```python
from build123d import *

# Parameters (mm, degrees)
F0_R     = 122.5
F0_R_2   = 3
F1_DEPTH = 16.5
F4_R     = 1


with BuildPart() as f1:
    # F0 (on Front) → F1 (new body)
    with BuildSketch(Plane.XZ):
        Circle(F0_R)
        with Locations((-81.31728, -81.31728)):
            Circle(F0_R_2, mode=Mode.SUBTRACT)
        with Locations((0, -115)):
            Circle(F0_R_2, mode=Mode.SUBTRACT)
        with Locations((81.31728, -81.31728)):
            Circle(F0_R_2, mode=Mode.SUBTRACT)
        with Locations((-115, 0)):
            Circle(F0_R_2, mode=Mode.SUBTRACT)
        with Locations((-81.31728, 81.31728)):
            Circle(F0_R_2, mode=Mode.SUBTRACT)
        with BuildLine():
            ThreePointArc((-99.728162, 7.368421), (-70.710678, 70.710678), (-7.368421, 99.728162))
            ThreePointArc((-7.368421, 99.728162), (0, 100), (7.368421, 99.728162))
            ThreePointArc((7.368421, 99.728162), (70.710678, 70.710678), (99.728162, 7.368421))
            ThreePointArc((99.728162, 7.368421), (99.932017, 3.686717), (100, 0))
            ThreePointArc((100, 0), (99.932017, -3.686717), (99.728162, -7.368421))
            ThreePointArc((99.728162, -7.368421), (70.710678, -70.710678), (7.368421, -99.728162))
            ThreePointArc((7.368421, -99.728162), (0, -100), (-7.368421, -99.728162))
            ThreePointArc((-7.368421, -99.728162), (-70.710678, -70.710678), (-99.728162, -7.368421))
            ThreePointArc((-99.728162, -7.368421), (-100, 0), (-99.728162, 7.368421))
        make_face(mode=Mode.SUBTRACT)
        with Locations((115, 0)):
            Circle(F0_R_2, mode=Mode.SUBTRACT)
        with Locations((0, 115)):
            Circle(F0_R_2, mode=Mode.SUBTRACT)
        with Locations((81.31728, 81.31728)):
            Circle(F0_R_2, mode=Mode.SUBTRACT)
    extrude(amount=F1_DEPTH)

    # F2 (on Right) → F3 (revolve, cut)
    with BuildSketch(Plane.YZ):
        Polygon((-12.5, 104), (-4, 104), (-4, 126.782835), (-12.5, 127.067506), align=None)
    revolve(axis=Axis((0, 30.039648, 0), (0, 1, 0)), mode=Mode.SUBTRACT)

    # F4
    f4_edges = [f1.edges().sort_by_distance(p)[0] for p in [
        (-122.5, -16.5, 0),
        (-122.5, 0, 0),
    ]]
    fillet(f4_edges, radius=F4_R)


solid = f1.part
```
For this review, take the finished solid that the model builds, in its own axes (mm). A direction names the side the tool comes from. Coordinates: 2 decimals unless noted, no trailing zeros. Order: outer loops, then holes, each group sorted by start corner. A loop starts at its lowest first (then second) coordinate and runs counter-clockwise, first axis right, second up. Notation, with made-up numbers: (57, 45) -> (80, 45) arc R9 cw to (80, 61) -> close; hole circle Ø6 at (2.25, -9.5). An arc over 180 degrees is marked (long way). Answer as CSV lines item,"result".
Q1. We need section A-A (y = -9.25). State the section outline as (x, z) points.
Model answer:
outline,"circle Ø208 at (0, 0); hole (-99.73, -7.37) arc R100 ccw to (-7.37, -99.73) arc R100 ccw to (7.37, -99.73) arc R100 ccw to (99.73, -7.37) arc R100 ccw to (100, 0) arc R100 ccw to (99.73, 7.37) arc R100 ccw to (7.37, 99.73) arc R100 ccw to (-7.37, 99.73) arc R100 ccw to (-99.73, 7.37) arc R100 ccw to start"
Q2. Clearance check with flat-ended pins moving along their axes: pin 1 Ø3.5 at (x, z) = (81.32, -81.32) entering from +Y; pin 2 Ø2 at (x, y) = (89.5, -10) entering from -Z; pin 3 Ø5 at (x, y) = (57.5, -5.5) entering from +Z. State where each tip first meets the part, or that it passes through.
Model answer:
pin 1,"passes through"
pin 2,"stops at z = -54.62"
pin 3,"stops at z = 109.21"
Q3. For faces 5 (the face through (27.8, -12.5, -100.4)), 6 (the face through (-91, 0, -44)), 7 (the face through (0, -8, -100)), list the 3-axis set-ups (+Z, -Z, +X, -X, +Y, -Y) from which the entire face can be reached by the end or side of a thin tool; tool diameter is ignored.
Model answer:
face 5,"none"
face 6,"+Z, -Z, +X, -X, +Y"
face 7,"+Y, -Y"
Q4. We need section B-B (x = -115). Count the separate pieces of the cut face and the enclosed holes in it, plus the area to 3 significant figures.
Model answer:
separate pieces,"4"
enclosed holes,"0"
area,"625 mm2"
Q5. Draft analysis for pull direction Z (two halves, no side actions). For faces 1 (the face through (-83.528, -1.972, 83.345)), 2 (the face through (-63.282, -8.19, -82.531)), 3 (the face through (-112.14, -14.47, 0.9)), 4 (the face through (-91, -16.5, -44)), state which applies: released by +Z, released by -Z, zero draft, split by the parting line, or undercut.
Model answer:
face 1,"undercut"
face 2,"split by the parting line"
face 3,"undercut"
face 4,"zero draft"
Q6. Wall thickness on line 1 along Y through (x, z) = (38.5, -97); line 2 along Z through (x, y) = (-0.5, -12.25); line 3 along X through (y, z) = (-11, 80): over which ranges is each line inside the solid? List them lowest first. Write a range as [from, to].
Model answer:
line 1,"y = [-16.5, -12.5], [-4, 0]"
line 2,"z = [-104, -100], [100, 104]"
line 3,"x = [-66.45, -60], [60, 66.45]"
